Work out the finished part from the listing and answer in its coordinate system (mm). Coordinates: 2 decimals unless noted, no trailing zeros. Order: outer loops, then holes, each group sorted by start corner. A loop starts at its lowest first (then second) coordinate and runs counter-clockwise, first axis right, second up. Notation, with made-up numbers: M 70.25,52.25 L 114.25,52.25 A22 cw 114.25,65.25 Z; hole C 64,76.5 d6. An arc over 180 degrees is marked long. Answer in a Markdown table with one row per item. Add a question column.
Item 1: The part is cut by section B-B (y = 13). Write down the section's boundary in (x, z) (3 decimals).
Item 2: Flat-ended cylindrical pins translate along their axes: pin 1 Ø3 at (x, z) = (-90.5, -7) entering from -Y; pin 2 Ø12 at (y, z) = (17.5, 12) entering from +X; pin 3 Ø1 at (x, z) = (-22.5, -3) entering from -Y. Find the tip coordinate at first contact, or state that the pin passes through.
Item 3: Consider line 1 (Y direction, x = -102, z = -17); line 2 (Z direction, x = 39, y = 19.5); line 3 (Z direction, x = -52, y = 20). Determine where each line is inside the solid, lowest interval first. Write a range as from..to.
Item 4: The mould has two halves that part along Z. Classify faces 1 (the face through (-1.78, 4.76, -0.15)), 2 (the face through (-123.38, 27.93, -0.04)), 3 (the face through (-1, 9, -28.575)), 4 (the face through (-119.757, 9.392, 20.937)): released by +Z, released by -Z, zero draft, split by the parting line, or undercut.
from build123d import *

# Parameters (mm, degrees)
SKETCH1_W               = 254
SKETCH1_H               = 57.15
BOSS_EXTRUDE1_DEPTH     = 31.75
FILLET1_R               = 12.7
FILLET2_R               = 25.4
CUT_EXTRUDE1_DEPTH      = 134.991018822
CUT_EXTRUDE1_DEPTH_BACK = 134.991018822
SKETCH2_R               = 11.1125


with BuildPart() as part:
    # Sketch1 → Boss-Extrude1 (new body)
    with BuildSketch(Plane(origin=(0, 0, 0), x_dir=(1, 0, 0), z_dir=(0, 1, 0))):
        Rectangle(SKETCH1_W, SKETCH1_H)
    extrude(amount=BOSS_EXTRUDE1_DEPTH)

    # Fillet1
    fillet1_edges = [part.edges().sort_by_distance(p)[0] for p in [
        (-127, 31.75, 0),
        (0, 31.75, 28.575),
        (127, 31.75, 0),
        (0, 31.75, -28.575),
    ]]
    fillet(fillet1_edges, radius=FILLET1_R)

    # Fillet2
    # the kernel refuses this fillet: 25.4 mm, written as the material it takes off along each edge
    with BuildSketch(Plane(origin=(101.6, 31.75, -3.175), x_dir=(1, 0, 0), z_dir=(0, 0, 1))) as fillet2_piece_1:
        with BuildLine():
            CenterArc((12.7, -12.7), 12.7, 0, 90)
            Line((25.4, -12.7), (25.4, 0))
            Line((25.4, 0), (12.7, 0))
        make_face()
    revolve(axis=Axis((101.6, 31.75, -3.175), (0, 1, 0)), revolution_arc=90, mode=Mode.SUBTRACT)
    with BuildSketch(Plane(origin=(101.6, 31.75, 3.175), x_dir=(0, 0, 1), z_dir=(-1, 0, 0))) as fillet2_piece_2:
        with BuildLine():
            CenterArc((12.7, -12.7), 12.7, 0, 90)
            Line((25.4, -12.7), (25.4, 0))
            Line((25.4, 0), (12.7, 0))
        make_face()
    revolve(axis=Axis((101.6, 31.75, 3.175), (0, 1, 0)), revolution_arc=90, mode=Mode.SUBTRACT)
    with BuildSketch(Plane(origin=(-101.6, 31.75, -3.175), x_dir=(0, 0, -1), z_dir=(1, 0, 0))) as fillet2_piece_3:
        with BuildLine():
            CenterArc((12.7, -12.7), 12.7, 0, 90)
            Line((25.4, -12.7), (25.4, 0))
            Line((25.4, 0), (12.7, 0))
        make_face()
    revolve(axis=Axis((-101.6, 31.75, -3.175), (0, 1, 0)), revolution_arc=90, mode=Mode.SUBTRACT)
    with BuildSketch(Plane(origin=(-101.6, 31.75, 3.175), x_dir=(-1, 0, 0), z_dir=(0, 0, -1))) as fillet2_piece_4:
        with BuildLine():
            CenterArc((12.7, -12.7), 12.7, 0, 90)
            Line((25.4, -12.7), (25.4, 0))
            Line((25.4, 0), (12.7, 0))
        make_face()
    revolve(axis=Axis((-101.6, 31.75, 3.175), (0, 1, 0)), revolution_arc=90, mode=Mode.SUBTRACT)
    with BuildSketch(Plane(origin=(-127, -63.5, 28.575), x_dir=(0, 0, -1), z_dir=(0, 1, 0)), Plane(origin=(-127, -63.5, -28.575), x_dir=(1, 0, 0), z_dir=(0, 1, 0))) as fillet2_piece_5:
        with BuildLine():
            CenterArc((FILLET2_R, -FILLET2_R), FILLET2_R, 90, 90)
            Line((0, -FILLET2_R), (0, 0))
            Line((0, 0), (FILLET2_R, 0))
        make_face()
    extrude(amount=95.25, mode=Mode.SUBTRACT)
    with BuildSketch(Plane(origin=(127, -63.5, -28.575), x_dir=(-1, 0, 0), z_dir=(0, 1, 0)), Plane(origin=(127, -63.5, 28.575), x_dir=(0, 0, -1), z_dir=(0, 1, 0))) as fillet2_piece_6:
        with BuildLine():
            CenterArc((FILLET2_R, FILLET2_R), FILLET2_R, 180, 90)
            Line((0, FILLET2_R), (0, 0))
            Line((0, 0), (FILLET2_R, 0))
        make_face()
    extrude(amount=95.25, mode=Mode.SUBTRACT)

    # Sketch2 → Cut-Extrude1 (cut, two sides: drawn at the far end of the back side and taken through both)
    with BuildSketch(Plane(origin=(0, 0, 0), x_dir=(0, 0, -1), z_dir=(1, 0, 0)).offset(-CUT_EXTRUDE1_DEPTH_BACK)):
        with Locations((0, -6.35)):
            Circle(SKETCH2_R)
    extrude(amount=CUT_EXTRUDE1_DEPTH + CUT_EXTRUDE1_DEPTH_BACK, mode=Mode.SUBTRACT)


solid = part.part
Reply:
| question | item | result |
|---|---|---|
| 1 | outline | M -127,-3.175 A25.4 ccw -101.6,-28.575 L 101.6,-28.575 A25.4 ccw 127,-3.175 L 127,3.175 A25.4 ccw 101.6,28.575 L -101.6,28.575 A25.4 ccw -127,3.175 Z |
| 2 | pin 1 | stops at y = 0.81 |
| 2 | pin 2 | stops at x = 126.84 |
| 2 | pin 3 | stops at y = 4.2 |
| 3 | line 1 | y = 0..31.7 |
| 3 | line 2 | z = -28.57..28.57 |
| 3 | line 3 | z = -28.54..28.54 |
| 4 | face 1 | undercut |
| 4 | face 2 | zero draft |
| 4 | face 3 | released by -Z |
| 4 | face 4 | released by +Z |
